```python
from build123d import *

# Parameters (mm, degrees)
SKETCH1_R                       = 11
SKETCH1_R_2                     = 5.1
BOSS_EXTRUDE1_DEPTH             = 10
SKETCH2_R                       = 1.75
CUT_EXTRUDE1_DEPTH              = 19.493242009
BOSS_EXTRUDE2_START             = 11
SKETCH3_W                       = 22
SKETCH3_H                       = 10
BOSS_EXTRUDE2_DEPTH             = 10.16
BOSS_EXTRUDE3_REACH             = 28.552
SKETCH5_W                       = 22
SKETCH5_H                       = 10
SKETCH6_W                       = 10.16
SKETCH6_H                       = 13.97
CUT_EXTRUDE2_DEPTH              = 26.860116009
SKETCH7_R                       = 1.75
CUT_EXTRUDE3_DEPTH              = 33.120797001
BOSS_EXTRUDE4_DEPTH             = 10
BOSS_EXTRUDE5_REACH             = 27.86
SKETCH9_W                       = 10
SKETCH9_H                       = 0.75
BOSS_EXTRUDE5_DIRECTION_2_REACH = 27.86
BOSS_EXTRUDE6_DEPTH             = 1.25
FILLET1_R                       = 1.5


with BuildPart() as part:
    # Sketch1 → Boss-Extrude1 (new body)
    with BuildSketch(Plane.XY):
        Circle(SKETCH1_R)
        Circle(SKETCH1_R_2, mode=Mode.SUBTRACT)
    extrude(amount=BOSS_EXTRUDE1_DEPTH)

    # Sketch2 → Cut-Extrude1 (cut, through all)
    with BuildSketch(Plane.XY.offset(10)):
        with Locations((0, 8)):
            Circle(SKETCH2_R)
        with Locations((8, 0)):
            Circle(SKETCH2_R)
        with Locations((0, -8)):
            Circle(SKETCH2_R)
        with Locations((-8, 0)):
            Circle(SKETCH2_R)
    extrude(amount=-CUT_EXTRUDE1_DEPTH, mode=Mode.SUBTRACT)

    # Sketch5 → Boss-Extrude3 (add, up to next)
    with BuildSketch(Plane.XZ.offset(-11), mode=Mode.PRIVATE) as boss_extrude3_sk1:
        with Locations((0, 5)):
            Rectangle(SKETCH5_W, SKETCH5_H)
    boss_extrude3_tool1 = extrude(boss_extrude3_sk1.sketch, amount=BOSS_EXTRUDE3_REACH, mode=Mode.PRIVATE) - part.part


with BuildPart() as body_2:
    # Sketch3 → Boss-Extrude2 (new body)
    with BuildSketch(Plane(origin=(0, 0, 0), x_dir=(1, 0, 0), z_dir=(0, 1, 0)).offset(BOSS_EXTRUDE2_START)):
        with Locations((0, -5)):
            Rectangle(SKETCH3_W, SKETCH3_H)
    extrude(amount=BOSS_EXTRUDE2_DEPTH)


with BuildPart() as part_1:
    add(part.part)

    add(body_2.part)  # Boss-Extrude3 merges body 2
    add(boss_extrude3_tool1.solids().sort_by_distance((0, 11, 5))[0])
    add(boss_extrude3_tool1.solids().sort_by_distance((0, 11, 5))[1])

    # Sketch6 → Cut-Extrude2 (cut, through all)
    with BuildSketch(Plane.XY.offset(10)):
        with Locations((0, 14.175)):
            Rectangle(SKETCH6_W, SKETCH6_H)
    extrude(amount=-CUT_EXTRUDE2_DEPTH, mode=Mode.SUBTRACT)

    # Sketch7 → Cut-Extrude3 (cut, through all)
    with BuildSketch(Plane(origin=(11, 0, 0), x_dir=(0, 0, -1), z_dir=(1, 0, 0))):
        with Locations((-5, 16.08)):
            Circle(SKETCH7_R)
    extrude(amount=-CUT_EXTRUDE3_DEPTH, mode=Mode.SUBTRACT)

    # Sketch8 → Boss-Extrude4 (add, through all)
    with BuildSketch(Plane.XY.offset(10)):
        with BuildLine():
            Line((-11, 0), (-11, -11))
            Line((-11, -11), (-4.5e-08, -11))
            ThreePointArc((-4.5e-08, -11), (-7.778174609, -7.778174577), (-11, 0))
        make_face()
        with BuildLine():
            ThreePointArc((11, 0), (7.778174577, -7.778174609), (-4.5e-08, -11))
            Line((-4.5e-08, -11), (11, -11))
            Line((11, -11), (11, 0))
        make_face()
    extrude(amount=-BOSS_EXTRUDE4_DEPTH)

    # Sketch9 → Boss-Extrude5 (add, up to next)
    with BuildSketch(Plane.ZY, mode=Mode.PRIVATE) as boss_extrude5_sk1:
        with Locations((5, 10.485)):
            Rectangle(SKETCH9_W, SKETCH9_H)
    boss_extrude5_tool1 = extrude(boss_extrude5_sk1.sketch, amount=BOSS_EXTRUDE5_REACH, mode=Mode.PRIVATE) - part_1.part
    add(boss_extrude5_tool1.solids().sort_by_distance((0, 10.485, 5))[0])

    # Sketch9 → Boss-Extrude5 direction 2 (add, up to next)
    with BuildSketch(Plane.ZY, mode=Mode.PRIVATE) as boss_extrude5_direction_2_sk1:
        with Locations((5, 10.485)):
            Rectangle(SKETCH9_W, SKETCH9_H)
    boss_extrude5_direction_2_tool1 = extrude(boss_extrude5_direction_2_sk1.sketch, amount=-BOSS_EXTRUDE5_DIRECTION_2_REACH, mode=Mode.PRIVATE) - part_1.part
    add(boss_extrude5_direction_2_tool1.solids().sort_by_distance((0, 10.485, 5))[0])

    # Sketch10 → Boss-Extrude6 (add, symmetric)
    with BuildSketch(Plane.ZY):
        Polygon((5, 11.86), (3.267949192, 10.86), (6.732050808, 10.86), align=None)
    extrude(amount=BOSS_EXTRUDE6_DEPTH, both=True)

    # Fillet1
    fillet1_edges = [part_1.edges().sort_by_distance(p)[0] for p in [
        (0, 11.86, 5),
    ]]
    fillet(fillet1_edges, radius=FILLET1_R)


solid = part_1.part
```
Geometry check sheet. Reference: the model listing, model coordinates, mm. A direction names the side the tool comes from. Coordinates: 2 decimals unless noted, no trailing zeros. Order: outer loops, then holes, each group sorted by start corner. A loop starts at its lowest first (then second) coordinate and runs counter-clockwise, first axis right, second up. Notation, with made-up numbers: (47, 19.25) - (83, 19.25) arc R26 cw to (83, 53.25) - close; hole circle Ø9 at (-5, -16). An arc over 180 degrees is marked (long way). Answer in a Markdown table with one row per item. Add a question column.
1. Material ranges on L1, parallel to Y at x = 0, z = 3.5; L2, parallel to X at y = 11.5, z = 4.5; L3, parallel to X at y = 15, z = 8.25, recorded low to high. Write a range as [from, to].
2. Section check B-B (z = 5). Give the number of separate pieces and of enclosed holes in the cut face, plus the area to 3 significant figures.
3. Access from +Z, -Z, +X, -X, +Y, -Y to the whole of each face (thin tool, end or side, straight path). Record for faces 1 (the face through (5.08, 16, 7)), 2 (the face through (-0.02, 11.14, 6.25)), 3 (the face through (-0.02, 11.15, 3.77)), 4 (the face through (3, 7.19, 5)).
4. Section check D-D (x = 0). Enter the section's corners in (y, z).
5. Gauge pin test, flat ends, axial feed: pin 1 Ø1 at (x, y) = (-7.5, 11.5) entering from -Z; pin 2 Ø1.1 at (x, z) = (-3.5, 3.5) entering from +Y. Record the tip position at first contact, or that the pin passes through.
6. Draft check along X on faces 5 (the face through (0, 10.86, 7)), 6 (the face through (8.081, 17.815, 5.228)), 7 (the face through (11, 5, 5)). Enter one of: +X half, -X half, draft (parallel to the pull), parting line (faces both ways), or undercut.
7. Section check A-A (x = -8). Enter the section's corners in (y, z), plus the area to 3 significant figures.
8. Section check C-C (y = -8). Enter the section's corners in (x, z).
Data:
| question | item | result |
|---|---|---|
| 1 | L1 | y = [-11, -9.75], [-6.25, -5.1], [5.1, 6.25], [10.11, 10.99] |
| 1 | L2 | x = [-11, -5.08], [-1.25, 1.25], [5.08, 11] |
| 1 | L3 | x = [-11, -5.08], [5.08, 11] |
| 2 | separate pieces | 3 |
| 2 | enclosed holes | 5 |
| 2 | area | 421 mm² |
| 3 | face 1 | +Z, -Z, +Y |
| 3 | face 2 | +Z, +Y |
| 3 | face 3 | -Z, +Y |
| 3 | face 4 | +Z, -Z |
| 4 | outline | (-11, 0) - (-9.75, 0) - (-9.75, 10) - (-11, 10) - close; (-6.25, 0) - (-5.1, 0) - (-5.1, 10) - (-6.25, 10) - close; (5.1, 0) - (6.25, 0) - (6.25, 10) - (5.1, 10) - close; (10.11, 0) - (10.86, 0) - (10.86, 3.27) - (11.43, 4.25) arc R1.5 ccw to (11.43, 5.75) - (10.86, 6.73) - (10.86, 10) - (10.11, 10) - close |
| 5 | pin 1 | stops at z = 0 |
| 5 | pin 2 | stops at y = 10.86 |
| 6 | face 5 | undercut |
| 6 | face 6 | draft |
| 6 | face 7 | +X half |
| 7 | outline | (-11, 0) - (-1.75, 0) - (-1.75, 10) - (-11, 10) - close; (1.75, 0) - (21.16, 0) - (21.16, 10) - (1.75, 10) - close; hole circle Ø3.5 at (16.08, 5) |
| 7 | area | 277 mm² |
| 8 | outline | (-11, 0) - (-1.75, 0) - (-1.75, 10) - (-11, 10) - close; (1.75, 0) - (11, 0) - (11, 10) - (1.75, 10) - close |
